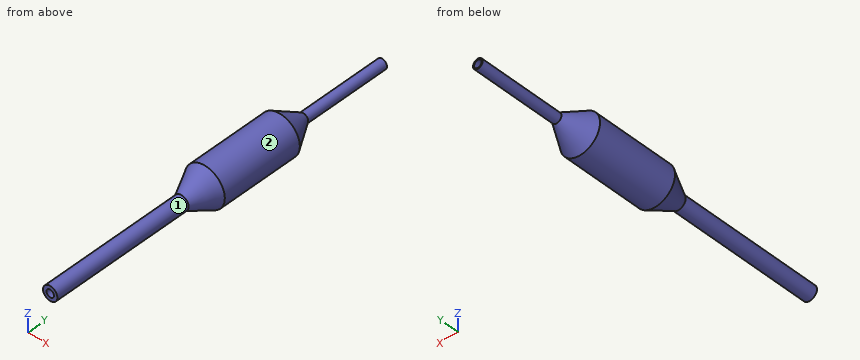
```python
from build123d import *

# Parameters (mm, degrees)
F2_R     = 0.9271
F3_DEPTH = 12.7
F4_R     = 0.9271
F5_DEPTH = 12.7


with BuildPart() as f1:
    # F0 (on Right) → F1 (revolve)
    with BuildSketch(Plane.YZ):
        Polygon((0, 1.778), (0, 0), (88.5, 0), (88.5, 1.2065), (67.5, 1.2065), (61.25, 4.9238), (41.25, 4.9238), (35, 1.778), align=None)
    revolve(axis=Axis((0, 44.25, 0), (0, 1, 0)))

    # F2 (on face) → F3 (cut)
    with BuildSketch(Plane(origin=(0, 88.5, 0), x_dir=(-1, 0, 0), z_dir=(0, 1, 0))):
        Circle(F2_R)
    extrude(amount=-F3_DEPTH, mode=Mode.SUBTRACT)

    # F4 (on face) → F5 (cut)
    with BuildSketch(Plane.XZ):
        Circle(F4_R)
    extrude(amount=-F5_DEPTH, mode=Mode.SUBTRACT)


solid = f1.part
```
Check sheet for the modelled part. Datum: model origin and axes. Units: mm. Face numbers are marked on the shaded views. A direction names the side the tool comes from. Round coordinates to 2 decimals unless told otherwise and drop trailing zeros. Write each loop counter-clockwise with the first axis right and the second up, starting at its lowest first coordinate (ties: lowest second). Pieces come first, ordered by that corner, then holes. Notation, with made-up numbers: (-14, -11.75) -> (16, -11.75) arc R14 cw to (16, 5.25) -> close; hole circle Ø4 at (-19.5, -35). An arc over 180 degrees is marked (long way). Put each result on its own line as item: value.
(1) Go/stop test with flat-tipped pins: pin 1 Ø4 at (x, z) = (3.5, 0) entering from +Y; pin 2 Ø0.6 at (x, z) = (0, -0.5) entering from -Y; pin 3 Ø1.5 at (y, z) = (64.5, 0) entering from -X. Record where each tip stops, or that it passes through.
Values found:
pin 1: stops at y = 67.01
pin 2: stops at y = 12.7
pin 3: stops at x = -3.44
(2) Material ranges on line 1 (X direction, y = 74.5, z = -0.75); line 2 (Y direction, x = -1.5, z = 1); line 3 (Y direction, x = 1.5, z = 0.25), recorded low to high.
Values found:
line 1: x = -0.95 to 0.95
line 2: y = 35.05 to 66.5
line 3: y = 0 to 66.97
(3) Tool access check on the marked faces 1 and 2. Record the directions out of +Z, -Z, +X, -X, +Y, -Y that give a thin tool (end or side, any length) a straight path to the whole face; none if there is none.
Values found:
face 1: -Y
face 2: +Y, -Y
(4) Sectioned sample at A-A (x = 0). Enter the section's corners in (y, z).
Values found:
outline: (0, -1.78) -> (35, -1.78) -> (41.25, -4.92) -> (61.25, -4.92) -> (67.5, -1.21) -> (88.5, -1.21) -> (88.5, -0.93) -> (75.8, -0.93) -> (75.8, 0.93) -> (88.5, 0.93) -> (88.5, 1.21) -> (67.5, 1.21) -> (61.25, 4.92) -> (41.25, 4.92) -> (35, 1.78) -> (0, 1.78) -> (0, 0.93) -> (12.7, 0.93) -> (12.7, -0.93) -> (0, -0.93) -> close
(5) Sectioned sample at C-C (y = 25). Enter the section's corners in (x, z), plus the area to 3 significant figures.
Values found:
outline: circle Ø3.56 at (0, 0)
area: 9.93 mm^2
(6) Sectioned sample at B-B (z = 0). Enter the section's corners in (x, y), plus the area to 3 significant figures.
Values found:
outline: (-4.92, 41.25) -> (-1.78, 35) -> (-1.78, 0) -> (-0.93, 0) -> (-0.93, 12.7) -> (0.93, 12.7) -> (0.93, 0) -> (1.78, 0) -> (1.78, 35) -> (4.92, 41.25) -> (4.92, 61.25) -> (1.21, 67.5) -> (1.21, 88.5) -> (0.93, 88.5) -> (0.93, 75.8) -> (-0.93, 75.8) -> (-0.93, 88.5) -> (-1.21, 88.5) -> (-1.21, 67.5) -> (-4.92, 61.25) -> close
area: 405 mm^2
